from build123d import *

# Parameters (mm, degrees)
SKETCH1_R           = 250
SKETCH1_R_2         = 162.5
BOSS_EXTRUDE1_DEPTH = 9.5
SKETCH2_R           = 213.5
SKETCH2_R_2         = 202.5
CUT_EXTRUDE1_DEPTH  = 7
SKETCH3_R           = 5
CUT_EXTRUDE2_DEPTH  = 355.063553617


with BuildPart() as part:
    # Sketch1 → Boss-Extrude1 (new, symmetric)
    with BuildSketch(Plane(origin=(0, 0, 0), x_dir=(1, 0, 0), z_dir=(0, 1, 0))):
        with Locations(Location((0, 0, 0), (0, 0, 270))):
            Circle(SKETCH1_R)
        with Locations(Location((0, 0, 0), (0, 0, 270))):
            Circle(SKETCH1_R_2, mode=Mode.SUBTRACT)
    extrude(amount=BOSS_EXTRUDE1_DEPTH, both=True)

    # Sketch2 → Cut-Extrude1 (cut)
    with BuildSketch(Plane(origin=(0, 9.5, 0), x_dir=(1, 0, 0), z_dir=(0, 1, 0))):
        with Locations(Location((0, 0, 0), (0, 0, 270))):
            Circle(SKETCH2_R)
        with Locations(Location((0, 0, 0), (0, 0, 270))):
            Circle(SKETCH2_R_2, mode=Mode.SUBTRACT)
    extrude(amount=-CUT_EXTRUDE1_DEPTH, mode=Mode.SUBTRACT)

    # Sketch3 → Cut-Extrude2 (cut, through all)
    with BuildSketch(Plane.XZ.offset(9.5)):
        with Locations(Location((111.25, 192.690652342, 0), (0, 0, 270))):
            Circle(SKETCH3_R)
        with Locations(Location((222.5, 0, 0), (0, 0, 270))):
            Circle(SKETCH3_R)
        with Locations(Location((-222.5, 0, 0), (0, 0, 90))):
            Circle(SKETCH3_R)
        with Locations(Location((-111.25, 192.690652342, 0), (0, 0, 90))):
            Circle(SKETCH3_R)
        with Locations(Location((-111.25, -192.690652342, 0), (0, 0, 270))):
            Circle(SKETCH3_R)
        with Locations(Location((111.25, -192.690652342, 0), (0, 0, 90))):
            Circle(SKETCH3_R)
    extrude(amount=-CUT_EXTRUDE2_DEPTH, mode=Mode.SUBTRACT)


solid = part.part
Build history of the part. All positions in model axes, mm. A direction names the side the tool comes from. Coordinates: 2 decimals unless noted, no trailing zeros. Order: outer loops, then holes, each group sorted by start corner. A loop starts at its lowest first (then second) coordinate and runs counter-clockwise, first axis right, second up. Notation, with made-up numbers: (-22, 62.25) - (35, 62.25) arc R19 ccw to (35, 77.25) - close; hole circle Ø1 at (6.25, -15). An arc over 180 degrees is marked (long way). Put each result on its own line as item: value.
1. Tool access for faces 1 (the face through (159, 2.5, 126)), 2 (the face through (186, 9.5, 110)): list every direction of +Z, -Z, +X, -X, +Y, -Y with a clear straight run to the whole face (end or side of a thin tool).
Answer sheet:
face 1: +Y
face 2: +Z, -Z, +X, -X, +Y
2. Saw through at C-C (z = 141.5). Write the cut outline in (x, y), and give its area (3 significant figures).
Answer sheet:
outline: (-206.1, -9.5) - (-79.9, -9.5) - (-79.9, 9.5) - (-144.86, 9.5) - (-144.86, 2.5) - (-159.87, 2.5) - (-159.87, 9.5) - (-206.1, 9.5) - close; (79.9, -9.5) - (206.1, -9.5) - (206.1, 9.5) - (159.87, 9.5) - (159.87, 2.5) - (144.86, 2.5) - (144.86, 9.5) - (79.9, 9.5) - close
area: 4,590 mm^2
3. Drop flat-ended pins along their axis: P1, Ø8, axis at x = 111.25, z = 192.69, coming from the -Y side; P2, Ø10, axis at x = -168.5, y = 4.5, coming from the +Z side; P3, Ø3, axis at y = 6.5, z = 52, coming from the +X side; P4, Ø1.5, axis at x = -17.5, y = -2.5, coming from the +Z side. Give the stop position or say it passes through.
Answer sheet:
P1: passes through
P2: stops at z = 189.12
P3: stops at x = 244.85
P4: stops at z = 249.44
4. Saw through at A-A (x = 0). Write the cut outline in (y, z), and give its area (3 significant figures).
Answer sheet:
outline: (-9.5, -250) - (9.5, -250) - (9.5, -213.5) - (2.5, -213.5) - (2.5, -202.5) - (9.5, -202.5) - (9.5, -162.5) - (-9.5, -162.5) - close; (-9.5, 162.5) - (9.5, 162.5) - (9.5, 202.5) - (2.5, 202.5) - (2.5, 213.5) - (9.5, 213.5) - (9.5, 250) - (-9.5, 250) - close
area: 3,170 mm^2
5. Probe line 1 along X through (y, z) = (7.5, 0); line 2 along X through (y, z) = (-5.25, 0); line 3 along X through (y, z) = (6.25, 92.5). List the from-to ranges inside material, lowest first. Write a range as [from, to].
Answer sheet:
line 1: x = [-250, -227.5], [-217.5, -213.5], [-202.5, -162.5], [162.5, 202.5], [213.5, 217.5], [227.5, 250]
line 2: x = [-250, -227.5], [-217.5, -162.5], [162.5, 217.5], [227.5, 250]
line 3: x = [-232.26, -192.42], [-180.14, -133.6], [133.6, 180.14], [192.42, 232.26]
6. Pull direction X, two halves, no side cores. Call faces 3 (the face through (61, 9.5, -151)), 4 (the face through (-197.685, 6.049, -43.898)), 5 (the face through (10.99, 0.13, -249.76)): pulls with the +X half, pulls with the -X half, needs draft (parallel to the pull), parting line crosses it, or undercut.
Answer sheet:
face 3: needs draft
face 4: undercut
face 5: parting line crosses it
7. Saw through at B-B (y = -5). Write the cut outline in (x, z).
Answer sheet:
outline: circle Ø500 at (0, 0); hole circle Ø10 at (-222.5, 0); hole circle Ø325 at (0, 0); hole circle Ø10 at (-111.25, -192.69); hole circle Ø10 at (-111.25, 192.69); hole circle Ø10 at (111.25, -192.69); hole circle Ø10 at (111.25, 192.69); hole circle Ø10 at (222.5, 0)
